Geometry check sheet. Reference: the model listing, model coordinates, mm. Give positions to 0.01 mm unless a question says otherwise; leave off trailing zeros. Write each loop counter-clockwise with the first axis right and the second up, starting at its lowest first coordinate (ties: lowest second). Pieces come first, ordered by that corner, then holes. Notation, with made-up numbers: (15, -9.75) -> (56, -9.75) arc R5 ccw to (56, -2.75) -> close; hole circle Ø7 at (11.25, 38.5). An arc over 180 degrees is marked (long way). Write item = value, one per line. Start each with the question number.
1. Cross-section at C-C, the plane y = 37.5. Record the cut outline in (x, z), plus the area to 3 significant figures.
2. Depth check by flat-ended pin: P1, Ø6, axis at x = 21.5, y = -10.5, coming from the -Z side; P2, Ø1.5, axis at y = 42.5, z = 1, coming from the -X side. Enter the tip coordinate at first touch or a pass-through.
3. Thickness scan on line 1 along X through (y, z) = (-48, 2.1); line 2 along Y through (x, z) = (13, 0.3); line 3 along X through (y, z) = (11.5, 0.3). Record the ranges inside material, lowest first.
4. Cross-section at A-A, the plane x = -34.5. State how many separate pieces and enclosed holes the cut face has, plus the area to 3 significant figures.
5. Cross-section at D-D, the plane y = 24. Record the cut outline in (x, z), plus the area to 3 significant figures.
```python
from build123d import *

# Parameters (mm, degrees)
F0_W     = 6
F0_H     = 3
F0_W_2   = 15
F0_W_3   = 7
F1_DEPTH = 3


with BuildPart() as f1:
    # F0 (on Top) → F1 (new body)
    with BuildSketch(Plane.XY):
        Polygon((-49.5, -52.5), (49.5, -52.5), (74.5, -52.5), (74.5, 52.5), (49.5, 52.5), (-40.5, 52.5), (-49.536567, 27.672236), (-54.188501, 1.289809), (-54.188501, -25.910191), align=None)
        Polygon((-40.172867, -47.809095), (-25.400751, -45.204372), (-24.879806, -48.158796), (-39.651922, -50.763518), align=None, mode=Mode.SUBTRACT)
        Polygon((-27.484529, -33.386679), (-42.256645, -35.991402), (-42.77759, -33.036979), (-28.005473, -30.432256), align=None, mode=Mode.SUBTRACT)
        with Locations((3, -46.704372)):
            Rectangle(F0_W, F0_H, mode=Mode.SUBTRACT)
        with Locations((-36.688501, -19.810191)):
            Rectangle(F0_W_2, F0_H, mode=Mode.SUBTRACT)
        with Locations((-36.688501, -4.810191)):
            Rectangle(F0_W_2, F0_H, mode=Mode.SUBTRACT)
        with Locations((13, -46.704372)):
            Rectangle(F0_W, F0_H, mode=Mode.SUBTRACT)
        with Locations((56, -18.369581)):
            Rectangle(F0_W_3, F0_H, mode=Mode.SUBTRACT)
        with Locations((67, -18.369581)):
            Rectangle(F0_W_3, F0_H, mode=Mode.SUBTRACT)
        Polygon((-43.056346, 6.835694), (-28.284229, 4.230971), (-28.805174, 1.276548), (-43.57729, 3.881271), align=None, mode=Mode.SUBTRACT)
        Polygon((-40.972567, 18.653387), (-40.451623, 21.60781), (-25.679507, 19.003088), (-26.200451, 16.048665), align=None, mode=Mode.SUBTRACT)
        Polygon((-22.137987, 29.854107), (-23.164047, 27.035029), (-37.259436, 32.165331), (-36.233376, 34.984409), align=None, mode=Mode.SUBTRACT)
        Polygon((-18.033745, 41.130419), (-32.129134, 46.260721), (-31.103074, 49.079799), (-17.007684, 43.949496), align=None, mode=Mode.SUBTRACT)
        with Locations((3, 42.630419)):
            Rectangle(F0_W, F0_H, mode=Mode.SUBTRACT)
        with Locations((13, 42.630419)):
            Rectangle(F0_W, F0_H, mode=Mode.SUBTRACT)
        with Locations((56, 42.630419)):
            Rectangle(F0_W_3, F0_H, mode=Mode.SUBTRACT)
        with Locations((67, 42.630419)):
            Rectangle(F0_W_3, F0_H, mode=Mode.SUBTRACT)
    extrude(amount=F1_DEPTH)


solid = f1.part
```
Answers:
q1.outline = (-45.96, 0) -> (74.5, 0) -> (74.5, 3) -> (-45.96, 3) -> close
q1.area = 361 mm^2
q2.P1 = 0
q2.P2 = -44.41
q3.line_1 = -50.29 to -40.14, -24.91 to 0, 6 to 10, 16 to 74.5
q3.line_2 = -52.5 to -48.2, -45.2 to 41.13, 44.13 to 52.5
q3.line_3 = -52.39 to 74.5
q4.separate_pieces = 8
q4.enclosed_holes = 0
q4.area = 251 mm^2
q5.outline = (-50.18, 0) -> (74.5, 0) -> (74.5, 3) -> (-50.18, 3) -> close
q5.area = 374 mm^2
